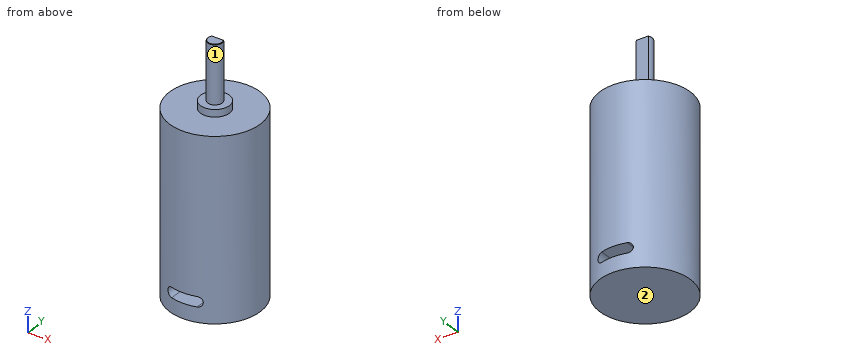
```python
from build123d import *

# Parameters (mm, degrees)
F2_W     = 3.4641016151
F2_H     = 1
F3_DEPTH = 12
F4_SIZE  = 0.127
F6_DEPTH = 76.2


with BuildPart() as f1:
    # F0 (on Right) → F1 (revolve)
    with BuildSketch(Plane.YZ):
        Polygon((0, 67.61), (0, 0), (12.5, 0), (12.5, 49.61), (4, 49.61), (4, 51.61), (2, 51.61), (2, 67.61), align=None)
    revolve(axis=Axis((0, 0, 33.805), (0, 0, -1)))

    # F2 (on face) → F3 (cut)
    with BuildSketch(Plane.XY.offset(67.61)):
        with Locations((0, 1.5)):
            Rectangle(F2_W, F2_H)
    extrude(amount=-F3_DEPTH, mode=Mode.SUBTRACT)

    # F4
    f4_edges = [f1.edges().sort_by_distance(p)[0] for p in [
        (0, -2, 67.61),
    ]]
    chamfer(f4_edges, length=F4_SIZE)

    # F5 (on Front) → F6 (cut, symmetric)
    with BuildSketch(Plane.XZ):
        with BuildLine():
            ThreePointArc((-2.1409534384, 5.472927049), (-2.5461377058, 6.4511284027), (-3.5243390594, 6.8563126701))
            Line((-3.5243390594, 6.8563126701), (-3.5243390594, 4.089541428))
            ThreePointArc((-3.5243390594, 4.089541428), (-2.5461377058, 4.4947256954), (-2.1409534384, 5.472927049))
        make_face()
        with BuildLine():
            Line((3.5243390594, 6.8563126701), (-3.5243390594, 6.8563126701))
            ThreePointArc((-3.5243390594, 6.8563126701), (-2.5461377058, 6.4511284027), (-2.1409534384, 5.472927049))
            ThreePointArc((-2.1409534384, 5.472927049), (-2.5461377058, 4.4947256954), (-3.5243390594, 4.089541428))
            Line((-3.5243390594, 4.089541428), (3.5243390594, 4.089541428))
            ThreePointArc((3.5243390594, 4.089541428), (2.1409534384, 5.472927049), (3.5243390594, 6.8563126701))
        make_face()
        with BuildLine():
            Line((-3.5243390594, 4.089541428), (-3.5243390594, 6.8563126701))
            ThreePointArc((-3.5243390594, 6.8563126701), (-4.9077246804, 5.472927049), (-3.5243390594, 4.089541428))
        make_face()
        with BuildLine():
            ThreePointArc((4.9077246804, 5.472927049), (4.502540413, 6.4511284027), (3.5243390594, 6.8563126701))
            Line((3.5243390594, 6.8563126701), (3.5243390594, 4.089541428))
            ThreePointArc((3.5243390594, 4.089541428), (4.502540413, 4.4947256954), (4.9077246804, 5.472927049))
        make_face()
        with BuildLine():
            Line((3.5243390594, 4.089541428), (3.5243390594, 6.8563126701))
            ThreePointArc((3.5243390594, 6.8563126701), (2.1409534384, 5.472927049), (3.5243390594, 4.089541428))
        make_face()
    extrude(amount=F6_DEPTH, both=True, mode=Mode.SUBTRACT)


solid = f1.part
```
Model file for the job. Use its own axes, mm. Face numbers are marked on the shaded views. A direction names the side the tool comes from. Round coordinates to 2 decimals unless told otherwise and drop trailing zeros. Loops run counter-clockwise (first coordinate to the right, second up) from the corner with the lowest first, then second, coordinate; pieces in that order, holes last. Notation, with made-up numbers: M 61,49 L 88,49 A28 ccw 88,84 Z; hole C 12.5,-27.5 d5. An arc over 180 degrees is marked long. Put each result on its own line as item: value. Start each with the question number.
Item 1: Cut at D-D (y = -5.5). List the corners of the cut face in (x, z), then the cut area to 3 significant figures.
Item 2: Cut at C-C (z = 31). List the corners of the cut face in (x, y).
Item 3: 3-axis set-ups, long thin cutter, end or side, ignore diameter. For the marked faces 1 and 2: which of +Z, -Z, +X, -X, +Y, -Y reach the whole face in a straight line?
Item 4: Cut at A-A (x = 0). List the corners of the cut face in (y, z), then the cut area to 3 significant figures.
Item 5: Drop flat-ended pins along their axis: P1, Ø4, axis at x = -1, z = 63, coming from the +Y side; P2, Ø2, axis at x = 8, y = 3, coming from the +Z side; P3, Ø8, axis at x = -9.5, z = 37.5, coming from the -Y side (3 decimals). Give the stop position or say it passes through.
Item 6: Drill centre lines: line 1 along Z through (x, y) = (-0.25, -0.75); line 2 along Z through (x, y) = (-2.5, 7.5); line 3 along Y through (x, z) = (-11.5, 35.5). Where is each one in solid material? Low to high.
Item 7: Cut at B-B (y = 0). List the corners of the cut face in (x, z), then the cut area to 3 significant figures.
Answer block:
1. outline: M -11.22,0 L 11.22,0 L 11.22,49.61 L -11.22,49.61 Z; hole M -3.52,4.09 L 3.52,4.09 A1.38 ccw 3.52,6.86 L -3.52,6.86 A1.38 ccw Z
1. area: 1,090 mm2
2. outline: C 0,0 d25
3. face 1: +Z
3. face 2: -Z, +X, -X, +Y, -Y
4. outline: M -12.5,0 L 12.5,0 L 12.5,4.09 L -12.5,4.09 Z; M -12.5,6.86 L 12.5,6.86 L 12.5,49.61 L 4,49.61 L 4,51.61 L 2,51.61 L 2,55.61 L 1,55.61 L 1,67.61 L -1.87,67.61 L -2,67.48 L -2,51.61 L -4,51.61 L -4,49.61 L -12.5,49.61 Z
4. area: 1,240 mm2
5. P1: y = 1
5. P2: z = 49.61
5. P3: y = -11.225
6. line 1: 0 to 4.09, 6.86 to 67.61
6. line 2: 0 to 4.09, 6.86 to 49.61
6. line 3: -4.9 to 4.9
7. outline: M -12.5,0 L 12.5,0 L 12.5,49.61 L 4,49.61 L 4,51.61 L 2,51.61 L 2,67.48 L 1.87,67.61 L -1.87,67.61 L -2,67.48 L -2,51.61 L -4,51.61 L -4,49.61 L -12.5,49.61 Z; hole M -3.52,4.09 L 3.52,4.09 A1.38 ccw 3.52,6.86 L -3.52,6.86 A1.38 ccw Z
7. area: 1,290 mm2
